Part model, mm, in its own coordinate system. A direction names the side the tool comes from. Coordinates: 2 decimals unless noted, no trailing zeros. Order: outer loops, then holes, each group sorted by start corner. A loop starts at its lowest first (then second) coordinate and runs counter-clockwise, first axis right, second up. Notation, with made-up numbers: (68, 66.5) - (83, 66.5) arc R29 ccw to (83, 87.5) - close; hole circle Ø4 at (-24.75, -7). An arc over 180 degrees is marked (long way). Use a Markdown table: item, result. Add a question column.
1) Tool access for faces 1 (the face through (60.517, 2.028, 55.76)), 2 (the face through (-63.01, 1.97, 32.85)), 3 (the face through (61.29, 1.97, -45.51)): list every direction of +Z, -Z, +X, -X, +Y, -Y with a clear straight run to the whole face (end or side of a thin tool).
2) Saw through at A-A on z = 62.5. List the corners of the cut face in (x, y).
3) Drop flat-ended pins along their axis: P1, Ø3.5, axis at x = -55.5, z = -62.53, coming from the +Y side; P2, Ø2, axis at x = 14, y = 1.5, coming from the -Z side; P3, Ø1.2, axis at x = -9, y = 3, coming from the +Z side. Give the stop position or say it passes through.
4) Saw through at D-D on y = 1.15. Count the separate pieces of the cut face and the enclosed holes in it, then the cut area to 3 significant figures.
5) Two-plate mould, pull along Z, no slides. Class faces 4 (the face through (77, 1.97, -27.18)), 5 (the face through (53.717, 2.028, -50.943)), 6 (the face through (1, 0, 1)): +Z half, -Z half, draft (parallel to the pull), parting line (faces both ways), or undercut.
6) Saw through at C-C on x = -29. List the corners of the cut face in (y, z), then the cut area to 3 significant figures.
7) Wall check: L1, parallel to X at y = 2.2, z = -61; L2, parallel to Z at x = 52.5, y = 2.4; L3, parallel to X at y = 2.65, z = 55.5. Give the ranges that are in metal, low to high. Write a range as [from, to].
8) Saw through at B-B on x = 62.5. List the corners of the cut face in (y, z), then the cut area to 3 significant figures.
Autodesk Inventor part; units mm, degrees
ref_plane "YZ Plane" through (0, 0, 0) normal (1, 0, 0) x (0, 1, 0)
ref_plane "XZ Plane" through (0, 0, 0) normal (0, 1, 0) x (-1, 0, 0)
ref_plane "XY Plane" through (0, 0, 0) normal (0, 0, 1) x (1, 0, 0)
sketch "Sketch1" plane through (0, 0, 0) normal (0, 1, 0) x (-1, 0, 0)
  line L0 (-0.0023, 59.9989) -> (-40.0023, 59.9989)
  line L1 (-0.0023, 59.9989) -> (39.9977, 59.9989) construction
  line L2 (-60.0163, -0.0152) -> (-60.0163, 39.9848)
  line L3 (-60.0163, -0.0152) -> (-20.0163, -0.0152) construction
  line L4 (-60.0163, -0.0152) -> (-0.0023, -0.0152)
  line L5 (-0.0023, -0.0152) -> (-0.0023, 59.9989)
  arc A0 (-49.9687, 64.958) -> (-40.0023, 59.9989) centre (-40.0023, 72.4933) ccw
  arc A1 (-60.0163, 39.9848) -> (-64.9755, 49.9513) centre (-72.5108, 39.9848) ccw
  arc A2 (-49.9687, 64.958) -> (-64.9755, 49.9513) centre (-58.5144, 58.4969) ccw
  line L6 (-40.0023, 59.9989) -> (-40.0023, 59.4989)
  line L7 (-60.0163, 39.9848) -> (-59.5163, 39.9848)
  arc A3 (-59.5163, 39.9848) -> (-40.0023, 59.4989) centre (-59.5163, 59.4989) ccw
  line L8 (-60.0163, -0.0152) -> (-80.0163, -0.0152)
  line L9 (-80.0163, -0.0152) -> (-80.0163, 19.9848)
  arc A4 (-70, 30.0011) -> (-60.0163, 39.9848) centre (-70, 39.9848) ccw
  arc A5 (-70, 30.0011) -> (-80.0163, 19.9848) centre (-70, 19.9848) ccw
  line L10 (-60.0163, -40.0152) -> (-59.5163, -40.0152)
  arc A6 (-64.9755, -49.9816) -> (-60.0163, -40.0152) centre (-72.5108, -40.0152) ccw
  line L11 (-60.0163, -0.0152) -> (-60.0163, -40.0152)
  arc A7 (-64.9755, -49.9816) -> (-49.9687, -64.9884) centre (-58.5144, -58.5273) ccw
  arc A8 (-40.0023, -60.0292) -> (-49.9687, -64.9884) centre (-40.0023, -72.5237) ccw
  arc A9 (-40.0023, -59.5292) -> (-59.5163, -40.0152) centre (-59.5163, -59.5292) ccw
  line L12 (-40.0023, -60.0292) -> (-40.0023, -59.5292)
  line L13 (-0.0023, -60.0292) -> (-40.0023, -60.0292)
  line L14 (-0.0023, -0.0152) -> (-0.0023, -60.0292)
  arc A10 (-60.0163, -40.0152) -> (-70, -30.0315) centre (-70, -40.0152) ccw
  line L15 (-80.0163, -0.0152) -> (-80.0163, -20.0152)
  arc A11 (-80.0163, -20.0152) -> (-70, -30.0315) centre (-70, -20.0152) ccw
  arc A12 (80.0118, 19.9848) -> (69.9955, 30.0011) centre (69.9955, 19.9848) ccw
  line L16 (60.0118, -0.0152) -> (80.0118, -0.0152)
  line L17 (80.0118, -0.0152) -> (80.0118, 19.9848)
  line L18 (-0.0023, 59.9989) -> (-40.0023, 59.9989) construction
  line L19 (-0.0023, 59.9989) -> (39.9977, 59.9989)
  line L20 (60.0118, -0.0152) -> (60.0118, 39.9848)
  arc A13 (60.0118, 39.9848) -> (69.9955, 30.0011) centre (69.9955, 39.9848) ccw
  line L21 (60.0118, 39.9848) -> (59.5118, 39.9848)
  arc A14 (64.9709, 49.9513) -> (60.0118, 39.9848) centre (72.5063, 39.9848) ccw
  line L22 (60.0118, -0.0152) -> (20.0118, -0.0152) construction
  arc A15 (64.9709, 49.9513) -> (49.9642, 64.958) centre (58.5098, 58.4969) ccw
  arc A16 (39.9977, 59.4989) -> (59.5118, 39.9848) centre (59.5118, 59.4989) ccw
  line L23 (39.9977, 59.9989) -> (39.9977, 59.4989)
  arc A17 (39.9977, 59.9989) -> (49.9642, 64.958) centre (39.9977, 72.4933) ccw
  line L24 (60.0118, -0.0152) -> (-0.0023, -0.0152)
  line L25 (80.0118, -0.0152) -> (80.0118, -20.0152)
  arc A18 (69.9955, -30.0315) -> (80.0118, -20.0152) centre (69.9955, -20.0152) ccw
  arc A19 (69.9955, -30.0315) -> (60.0118, -40.0152) centre (69.9955, -40.0152) ccw
  line L26 (60.0118, -40.0152) -> (59.5118, -40.0152)
  line L27 (60.0118, -0.0152) -> (60.0118, -40.0152)
  arc A20 (60.0118, -40.0152) -> (64.9709, -49.9816) centre (72.5063, -40.0152) ccw
  arc A21 (59.5118, -40.0152) -> (39.9977, -59.5292) centre (59.5118, -59.5292) ccw
  arc A22 (49.9642, -64.9884) -> (64.9709, -49.9816) centre (58.5098, -58.5273) ccw
  line L28 (39.9977, -60.0292) -> (39.9977, -59.5292)
  arc A23 (49.9642, -64.9884) -> (39.9977, -60.0292) centre (39.9977, -72.5237) ccw
  line L29 (-0.0023, -60.0292) -> (39.9977, -60.0292)
  point P0 (0, 0)
  point P1 (-55.5, 62.5)
  point P2 (-62.5, 55.5)
  point P3 (-52.5, 52.5)
  point P4 (-52.5, -52.5303)
  point P5 (-62.5, -55.5303)
  point P6 (-55.5, -62.5303)
  point P7 (55.4955, -62.5303)
  point P8 (62.4955, -55.5303)
  point P9 (52.4955, -52.5303)
  point P10 (52.4955, 52.5)
  point P11 (62.4955, 55.5)
  point P12 (55.4955, 62.5)
  point P13 (-65, 13.9848)
  point P14 (-65, -14.0152)
  dimension "d0" = 40
  dimension "d1" = 180
  dimension "d2" = 40
  dimension "d3" = 90
  dimension "d4" = 12.4944
  dimension "d5" = 12.4944
  dimension "d6" = 0.5
  dimension "d7" = 0.5
  dimension "d8" = 20
  dimension "d9" = 20
  dimension "d42" = 14
  dimension "d43" = 14
extrude "Extrusion1" add sketch "Sketch1" along normal blind 4 contours L5 L4 L2 L7 A3 L6 L0 | L19 L23 A16 L21 L20 L24 L5 | L14 L13 L12 A9 L10 L11 L4 | L24 L27 L26 A21 L28 L29 L14 | L8 L9 A5 A4 L2 | L11 A10 A11 L15 L8 | L20 A13 A12 L17 L16 | L16 L25 A18 A19 L27
extrude "Extrusion2" add sketch "Sketch1" along normal blind 4 contours L6 A3 L7 A1 A2 A0 | A17 A15 A14 L21 A16 L23 | L10 A9 L12 A8 A7 A6 | L28 A21 L26 A20 A22 A23
hole "Hole1" at (65, 0, -14.0152) direction (0, 1, 0) diameter 16.5 end through all
hole "Hole2" at (65, 0, 13.9848) direction (0, 1, 0) diameter 16.5 end through all
hole "Hole3" at (-55.4955, 0, 62.5) at (-62.4955, 0, 55.5) at (-52.4955, 0, 52.5) at (-52.4955, 0, -52.5303) at (-62.4955, 0, -55.5303) at (-55.4955, 0, -62.5303) at (55.5, 0, -62.5303) at (62.5, 0, -55.5303) at (52.5, 0, -52.5303) at (52.5, 0, 52.5) at (62.5, 0, 55.5) at (55.5, 0, 62.5) at (65, 0, 13.9848) at (65, 0, -14.0152) direction (0, 1, 0) diameter 4 end through all
properties part number "LowerPlatter" material "ABS Plastic"
Results are:
| question | item | result |
|---|---|---|
| 1 | face 1 | +Y, -Y |
| 1 | face 2 | -X, +Y, -Y |
| 1 | face 3 | +X, +Y, -Y |
| 2 | outline | (-68.45, 0) - (-57.5, 0) - (-57.5, 4) - (-68.45, 4) - close; (-53.5, 0) - (-47.5, 0) - (-47.5, 4) - (-53.5, 4) - close; (47.5, 0) - (53.5, 0) - (53.5, 4) - (47.5, 4) - close; (57.5, 0) - (68.45, 0) - (68.45, 4) - (57.5, 4) - close |
| 3 | P1 | through |
| 3 | P2 | z = -60.03 |
| 3 | P3 | z = 60 |
| 4 | separate pieces | 1 |
| 4 | enclosed holes | 14 |
| 4 | area | 17,200 mm2 |
| 5 | face 4 | -Z half |
| 5 | face 5 | undercut |
| 5 | face 6 | draft |
| 6 | outline | (0, -60.03) - (4, -60.03) - (4, 60) - (0, 60) - close |
| 6 | area | 480 mm2 |
| 7 | L1 | [-68.93, -56.78], [-54.21, -44.83], [44.83, 54.21], [56.79, 68.94] |
| 7 | L2 | [-67.39, -54.53], [-50.53, 50.5], [54.5, 67.36] |
| 7 | L3 | [-68.8, -64.5], [-60.5, 60.5], [64.5, 68.8] |
| 8 | outline | (0, -68.47) - (4, -68.47) - (4, -57.53) - (0, -57.53) - close; (0, -53.53) - (4, -53.53) - (4, -47.49) - (0, -47.49) - close; (0, -33.43) - (4, -33.43) - (4, -21.88) - (0, -21.88) - close; (0, -6.15) - (4, -6.15) - (4, 6.12) - (0, 6.12) - close; (0, 21.85) - (4, 21.85) - (4, 33.4) - (0, 33.4) - close; (0, 47.46) - (4, 47.46) - (4, 53.5) - (0, 53.5) - close; (0, 57.5) - (4, 57.5) - (4, 68.44) - (0, 68.44) - close |
| 8 | area | 277 mm2 |
